Build history of the part. All positions in model axes, mm. Face numbers are marked on the shaded views. A direction names the side the tool comes from. Give positions to 0.01 mm unless a question says otherwise; leave off trailing zeros. Loops run counter-clockwise (first coordinate to the right, second up) from the corner with the lowest first, then second, coordinate; pieces in that order, holes last. Notation, with made-up numbers: (73, 41) - (106, 41) arc R36 ccw to (106, 75) - close; hole circle Ø11 at (45, -10.75). An arc over 180 degrees is marked (long way). Return JSON: item names as keys, results as strings. Group by question number.
1) Slice it at B-B (x = -518.5). List the corners of the cut face in (y, z) (3 decimals).
2) 3-axis set-ups, long thin cutter, end or side, ignore diameter. For the marked faces 4 and 5: which of +Z, -Z, +X, -X, +Y, -Y reach the whole face in a straight line?
3) Drop flat-ended pins along their axis: pin 1 (3 mm diameter, centred on x = -577.5, z = -3, fed in from -Y); pin 2 (3 mm diameter, centred on y = 32, z = -3, fed in from -X); pin 3 (4 mm diameter, centred on x = -305, z = -309.5, fed in from -Y). Give the stop position or say it passes through.
4) Slice it at C-C (z = -415). List the corners of the cut face in (x, y), and give its area (3 significant figures).
5) Mould opens along Z. For the marked faces 1, 2 and 3 say: released by +Z, released by -Z, zero draft, split by the parting line, or undercut.
6) Slice it at A-A (y = 272). List the corners of the cut face in (x, z), and give its area (3 significant figures).
7) Drill centre lines: probe 1 along Z at (x, y) = (-113, 378.5); probe 2 along Y at (x, z) = (-433.5, -275.5). Where is each one in solid material? Low to high. Write a range as from..to.
8) Slice it at D-D (x = -181). List the corners of the cut face in (y, z) (3 decimals).
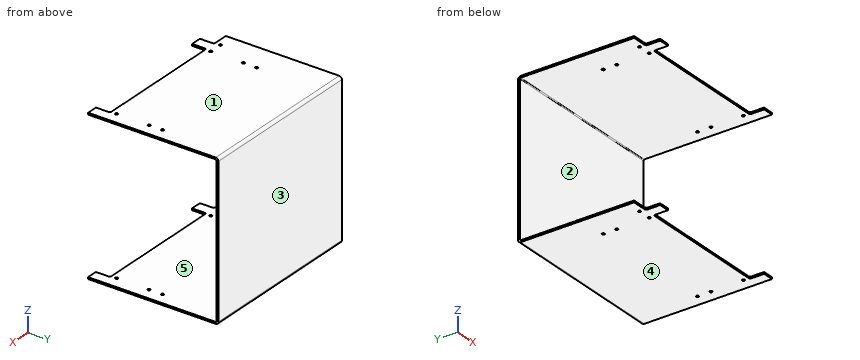
```python
from build123d import *

# Parameters (mm, degrees)
BOSS_EXTRUDE1_DEPTH          = 6.35
BOSS_EXTRUDE1_DEPTH_BACK     = 596.9
FILLET1_R                    = 3.175
FILLET2_R                    = 9.525
SKETCH2_W                    = 469.9
SKETCH2_H                    = 50.8
SKETCH2_W_2                  = 57.15
CUT_EXTRUDE1_DEPTH           = 547.1
FILLET3_R                    = 6.35
F_3_8_0_375_DIAMETER_HOLE1_D = 9.525


with BuildPart() as part:
    # Sketch1 → Boss-Extrude1 (new body, two sides)
    with BuildSketch(Plane(origin=(0, 0, 0), x_dir=(0, 0, -1), z_dir=(1, 0, 0))) as boss_extrude1_sk:
        Polygon((0, 0), (0, 463.55), (546.1, 463.55), (546.1, 0), (539.75, 0), (539.75, 457.2), (6.35, 457.2), (6.35, 0), align=None)
    extrude(amount=BOSS_EXTRUDE1_DEPTH)
    extrude(boss_extrude1_sk.sketch, amount=-BOSS_EXTRUDE1_DEPTH_BACK)

    # Fillet1
    fillet1_edges = [part.edges().sort_by_distance(p)[0] for p in [
        (-295.275, 457.2, -539.75),
        (-295.275, 457.2, -6.35),
    ]]
    fillet(fillet1_edges, radius=FILLET1_R)

    # Fillet2
    fillet2_edges = [part.edges().sort_by_distance(p)[0] for p in [
        (-295.275, 463.55, 0),
        (-295.275, 463.55, -546.1),
    ]]
    fillet(fillet2_edges, radius=FILLET2_R)

    # Sketch2 → Cut-Extrude1 (cut, through all)
    with BuildSketch(Plane.XY):
        with Locations((-266.7, 25.4)):
            Rectangle(SKETCH2_W, SKETCH2_H)
        with Locations((-568.325, 25.4)):
            Rectangle(SKETCH2_W_2, SKETCH2_H)
    extrude(amount=-CUT_EXTRUDE1_DEPTH, mode=Mode.SUBTRACT)

    # Fillet3
    fillet3_edges = [part.edges().sort_by_distance(p)[0] for p in [
        (-31.75, 50.8, -542.925),
        (-501.65, 50.8, -542.925),
        (-31.75, 50.8, -3.175),
        (-501.65, 50.8, -3.175),
        (-539.75, 50.8, -542.925),
        (-539.75, 50.8, -3.175),
    ]]
    fillet(fillet3_edges, radius=FILLET3_R)

    # 3/8 (0.375) Diameter Hole1 (through all)
    with Locations(Plane.XY):
        with Locations((-36.5125, 69.85), (-36.5125, 185.7375), (-36.5125, 233.3625), (-496.8875, 69.85), (-496.8875, 185.7375), (-496.8875, 233.3625), (-544.5125, 69.85)):
            Hole(F_3_8_0_375_DIAMETER_HOLE1_D / 2)


solid = part.part
```
Results:
{
 "1": {"outline": "(0, -546.1) - (454.025, -546.1) arc R9.525 ccw to (463.55, -536.575) - (463.55, -9.525) arc R9.525 ccw to (454.025, 0) - (0, 0) - (0, -6.35) - (454.025, -6.35) arc R3.175 cw to (457.2, -9.525) - (457.2, -536.575) arc R3.175 cw to (454.025, -539.75) - (0, -539.75) - close"},
 "2": {"face 4": "-Z, +X, -X, +Y, -Y", "face 5": "+X, -X, -Y"},
 "3": {"pin 1": "y = 50.8", "pin 2": "x = -539.75", "pin 3": "y = 457.2"},
 "4": {"outline": "(-596.9, 457.2) - (6.35, 457.2) - (6.35, 463.55) - (-596.9, 463.55) - close", "area": "3,830 mm2"},
 "5": {"face 1": "released by +Z", "face 2": "undercut", "face 3": "zero draft"},
 "6": {"outline": "(-596.9, -546.1) - (6.35, -546.1) - (6.35, -539.75) - (-596.9, -539.75) - close; (-596.9, -6.35) - (6.35, -6.35) - (6.35, 0) - (-596.9, 0) - close", "area": "7,660 mm2"},
 "7": {"probe 1": "-546.1..-539.75, -6.35..0", "probe 2": "457.2..463.55"},
 "8": {"outline": "(50.8, -546.1) - (454.025, -546.1) arc R9.525 ccw to (463.55, -536.575) - (463.55, -9.525) arc R9.525 ccw to (454.025, 0) - (50.8, 0) - (50.8, -6.35) - (454.025, -6.35) arc R3.175 cw to (457.2, -9.525) - (457.2, -536.575) arc R3.175 cw to (454.025, -539.75) - (50.8, -539.75) - close"}
}
